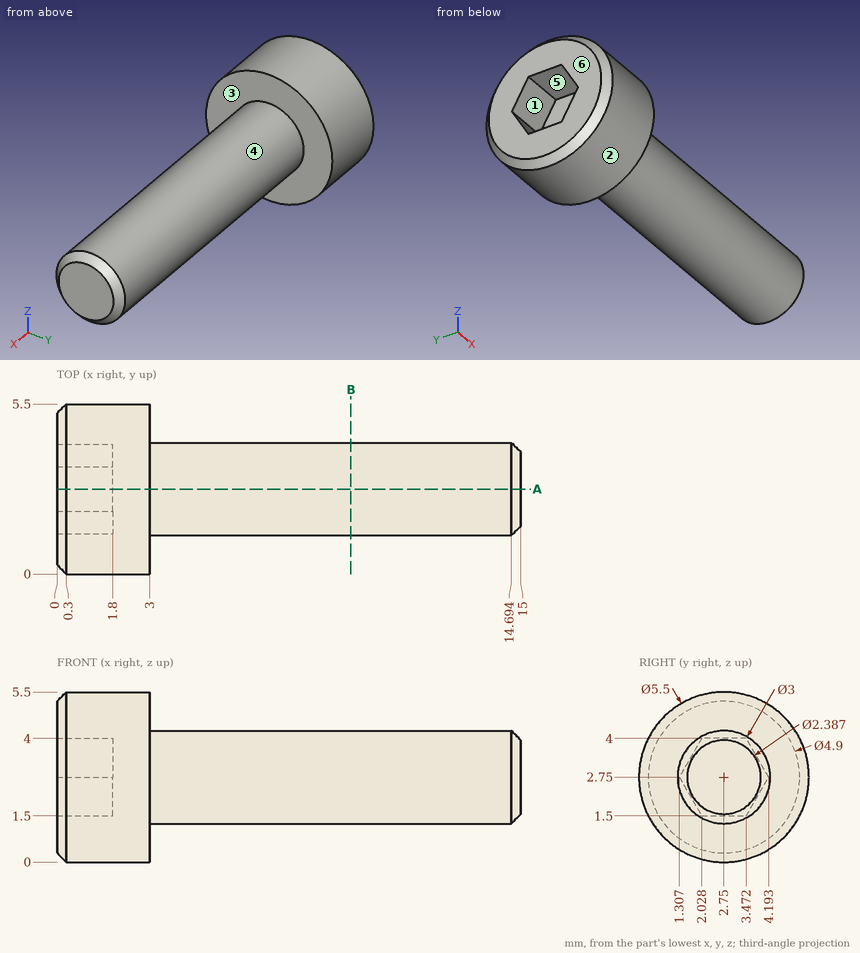
Design review of the part shown in the three views and the two pictorial views. Dimensions are in mm from the part's minimum x, y and z. A direction names the side the tool comes from. Round coordinates to 2 decimals unless told otherwise and drop trailing zeros. Loops run counter-clockwise (first coordinate to the right, second up) from the corner with the lowest first, then second, coordinate; pieces in that order, holes last. Notation, with made-up numbers: (-2, 35) -> (34, 35) arc R12 cw to (34, 55) -> close; hole circle Ø2 at (55, 41.5). An arc over 180 degrees is marked (long way). Answer as a JSON object with one key per item and string values. Group by question number.
1) For line 1 (X direction, y = 2.25, z = 4.5); line 2 (X direction, y = 2.5, z = 1.75); line 3 (Z direction, x = 10.75, y = 2.7), list the stretches that pass through material, from the lowest coordinate up. Write a range as [from, to].
2) For the marked faces 4, 5 and 6, list the 3-axis set-ups (+Z, -Z, +X, -X, +Y, -Y) from which the entire face can be reached by the end or side of a thin tool; tool diameter is ignored.
3) For pin 1 Ø1 at (x, y) = (2, 3.5) entering from +Z, flat-tipped, find the tip position at first contact; note if it passes through.
4) We need section A-A on y = 2.75. Write out the cut boundary in (x, z).
5) We need section B-B on x = 9.5. Write out the cut boundary in (y, z).
6) Mouldability with a two-part tool opening along Z and no side actions: class the marked faces 1, 2 and 3 as released by +Z, released by -Z, zero draft, split by the parting line, or undercut.
Result set:
{
 "1": {"line 1": "[0, 3]", "line 2": "[1.8, 15]", "line 3": "[1.25, 4.25]"},
 "2": {"face 4": "+X", "face 5": "-X", "face 6": "+Z, -Z, -X, +Y, -Y"},
 "3": {"pin 1": "z = 5.49"},
 "4": {"outline": "(0, 0.3) -> (0.3, 0) -> (3, 0) -> (3, 1.25) -> (14.69, 1.25) -> (15, 1.56) -> (15, 3.94) -> (14.69, 4.25) -> (3, 4.25) -> (3, 5.5) -> (0.3, 5.5) -> (0, 5.2) -> (0, 4) -> (1.8, 4) -> (1.8, 1.5) -> (0, 1.5) -> close"},
 "5": {"outline": "circle Ø3 at (2.75, 2.75)"},
 "6": {"face 1": "undercut", "face 2": "split by the parting line", "face 3": "zero draft"}
}
